Here's how the part is built. I have some questions about the finished solid (model axes, mm). A direction names the side the tool comes from. Round coordinates to 2 decimals unless told otherwise and drop trailing zeros. Loops run counter-clockwise (first coordinate to the right, second up) from the corner with the lowest first, then second, coordinate; pieces in that order, holes last. Notation, with made-up numbers: M 21,-15.5 L 71,-15.5 A25 ccw 71,23.5 Z; hole C 9,-11 d1. An arc over 180 degrees is marked long. Answer as a JSON object with one key per item and string values.
Autodesk Fusion 360 part; units mm, degrees
sketch "Sketch1" plane through (0, 0, 0) normal (0, 0, 1) x (1, 0, 0)
  line L0 (0, 0) -> (76.2, 0)
  line L1 (76.2, 0) -> (76.2, 146.05)
  line L2 (76.2, 146.05) -> (0, 146.05)
  line L3 (0, 146.05) -> (0, 0)
  line L4 (22.225, 0) -> (22.225, 146.05)
  line L5 (53.975, 146.05) -> (53.975, 0)
  line L6 (0, 133.35) -> (76.2, 133.35)
  line L7 (0, 114.3) -> (76.2, 114.3)
  line L8 (0, 60.325) -> (76.2, 60.325)
  line L9 (0, 47.625) -> (76.2, 47.625)
  dimension "d1" = 76.2
  dimension "d2" = 146.05
  dimension "d3" = 22.225
  dimension "d4" = 22.225
  dimension "d5" = 12.7
  dimension "d6" = 19.05
  dimension "d7" = 12.7
  dimension "d8" = 85.725
extrude "Extrude1" add sketch "Sketch1" against normal blind 12.7 contours L0 L3 L4 L9 | L0 L4 L5 L9 | L0 L1 L5 L9 makes body 1
extrude "Extrude2" add sketch "Sketch1" against normal blind 12.7 separate body contours L2 L3 L4 L6 | L2 L4 L5 L6 | L1 L2 L5 L6 makes body 2
extrude "Extrude3" add sketch "Sketch1" along normal blind 9.525 separate body contours L0 L4 L5 L9 | L4 L5 L8 L9 | L4 L5 L7 L8 | L4 L5 L6 L7 | L2 L4 L5 L6 makes body 3
extrude "Extrude4" add sketch "Sketch1" against normal blind 6.35 separate body contours L3 L4 L6 L7 | L4 L5 L6 L7 | L1 L5 L6 L7 makes body 4
extrude "Extrude5" add sketch "Sketch1" against normal blind 6.35 separate body contours L3 L4 L8 L9 | L4 L5 L8 L9 | L1 L5 L8 L9 makes body 5
extrude "Extrude6" add sketch "Sketch1" against normal blind 4.7625 separate body contours L3 L4 L7 L8 | L4 L5 L7 L8 | L1 L5 L7 L8 makes body 6
ref_plane "WorkPlane1" through (22.225, 146.05, 9.525) normal (0, 0, -1) x (-1, 0, 0)
sketch "Sketch2" plane through (22.225, 146.05, 9.525) normal (0, 0, -1) x (1, 0, 0)
  line L0 (53.975, 0) -> (-22.225, 0)
  line L1 (53.975, 146.05) -> (53.975, 0)
  line L2 (-22.225, 146.05) -> (53.975, 146.05)
  line L3 (-22.225, 0) -> (-22.225, 146.05)
  line L4 (9.525, 25.4) -> (9.525, 120.65)
  line L5 (22.225, 120.65) -> (22.225, 25.4)
  arc A0 (22.225, 120.65) -> (9.525, 120.65) centre (15.875, 120.65) ccw
  arc A1 (9.525, 25.4) -> (22.225, 25.4) centre (15.875, 25.4) ccw
  dimension "d21" = 12.7
  dimension "d22" = 12.7
  dimension "d23" = 25.4
  dimension "d24" = 25.4
  dimension "d25" = 38.1
  dimension "d26" = 38.1
  dimension "d27" = 6.35
  dimension "d28" = 6.35
ref_plane "WorkPlane2" through (38.1, 73.025, -1.5875) normal (0, 0, -1) x (1, 0, 0)
sketch "Sketch3" plane through (38.1, 73.025, -1.5875) normal (0, 0, -1) x (1, 0, 0)
  line L0 (-6.35, -47.625) -> (-6.35, 47.625)
  arc A0 (-6.35, -47.625) -> (6.35, -47.625) centre (0, -47.625) ccw
  line L1 (6.35, 47.625) -> (6.35, -47.625)
  arc A1 (6.35, 47.625) -> (-6.35, 47.625) centre (0, 47.625) ccw
  line L2 (-4.7625, -47.625) -> (-4.7625, 47.625)
  arc A2 (4.7625, 47.625) -> (-4.7625, 47.625) centre (0, 47.625) ccw
  line L3 (4.7625, 47.625) -> (4.7625, -47.625)
  arc A3 (-4.7625, -47.625) -> (4.7625, -47.625) centre (0, -47.625) ccw
  dimension "d30" = 1.5875
loft "Loft1" cut profiles "Sketch3", "Sketch2" section 1 contours L2 A2 L3 A3 section 2 contours L4 L5 A0 A1 bodies 1 3 4 5 6
combine "Combine1" operation add target body 1 tool bodies 2 3 4 5 6
fillet "Fillet1" radius 2 7 edges at (42.8625, 53.975, -1.5875) (42.8625, 36.5125, -1.5875) (33.3375, 28.0546, -1.5875) (33.3375, 53.975, -1.5875) (33.3375, 87.3125, -1.5875) (38.1, 125.4124, -1.5875) (42.8625, 87.3125, -1.5875) on bodies 1
Item 1: I want a section at B-B on y = 129. List the corners of the cut face in (x, z) for me (3 decimals), plus the area to 3 significant figures.
Solution:
{"outline": "M 0,-6.35 L 76.2,-6.35 L 76.2,0 L 53.975,0 L 53.975,9.525 L 22.225,9.525 L 22.225,0 L 0,0 Z", "area": "786 mm2"}
Item 2: I want a section at C-C on z = 8. List the corners of the cut face in (x, y) for me (3 decimals), plus the area to 3 significant figures.
Solution:
{"outline": "M 22.225,0 L 53.975,0 L 53.975,146.05 L 22.225,146.05 Z; hole M 31.968,25.4 A6.132 ccw 44.232,25.4 L 44.232,120.65 A6.132 ccw 31.968,120.65 Z", "area": "3,350 mm2"}
Item 3: We'd pull the mould along Y, two halves only. Please class faces 1 (the face through (22.225, 72, 5)), 2 (the face through (38, 88, -4.762)), 3 (the face through (39, 146.05, -4)): +Y half, -Y half, draft (parallel to the pull), parting line (faces both ways), or undercut.
Solution:
{"face 1": "draft", "face 2": "undercut", "face 3": "+Y half"}
Item 4: For P1, Ø5, axis at x = 35, y = 123.5, coming from the -Z side; P2, Ø3, axis at y = 66, z = 3, coming from the -X side (3 decimals); P3, Ø1, axis at x = 40, y = 101, coming from the -Z side, each with a flat end and sliding along its axis, tell me the tip position at first contact or that it passes through.
Solution:
{"P1": "stops at z = -6.35", "P2": "stops at x = 22.225", "P3": "stops at z = -4.76"}
Item 5: For faces 4 (the face through (38.225, 126.337, 4.893)), 5 (the face through (31, 74, 9.525)), 6 (the face through (53.975, 74, 5)), 7 (the face through (38, 54, -6.35)), 8 (the face through (76.2, 72, -3)), which set-ups out of +Z, -Z, +X, -X, +Y, -Y let a thin tool reach every point of the face, with its end or its side?
Solution:
{"face 4": "+Z", "face 5": "+Z, +X, -X, +Y, -Y", "face 6": "+Z, +X, +Y, -Y", "face 7": "-Z, +X, -X", "face 8": "+Z, -Z, +X, +Y, -Y"}
Item 6: If I drill on L1, parallel to Y at x = 55, z = -7.75 (3 decimals); L2, parallel to Z at x = 47.5, y = 79 (1 decimal); L3, parallel to Z at x = 16.5, y = 45, over which ranges is the centre line in solid material (lowest first)? Write a range as from..to.
Solution:
{"L1": "y = 0..47.625, 133.35..146.05", "L2": "z = -4.8..9.5", "L3": "z = -12.7..0"}
